Input: part model. Units: mm. Frame: model coordinates. A direction names the side the tool comes from. Round coordinates to 2 decimals unless told otherwise and drop trailing zeros. Loops run counter-clockwise (first coordinate to the right, second up) from the corner with the lowest first, then second, coordinate; pieces in that order, holes last.
(1) First-contact query: pin 1 Ø10 at (x, z) = (22.5, -40) entering from -Y. Flat tip, straight axial feed; report the tip coordinate or a pass-through.
(2) Cut plane B-B, the plane x = 22.5. Output: boundary loops of the cut face in (y, z).
(3) Draft query along Z for faces 1 (the face through (-97.5, -9, 1)), 2 (the face through (27.58, -8.88, -2.11)). Return one class per face: released by +Z, released by -Z, zero draft, split by the parting line, or undercut.
(4) Line query: line 1 (Z direction, x = -20, y = -7); line 2 (Z direction, x = 22.5, y = -6.5); line 3 (X direction, y = -16, z = -42). Output: solid intervals per line, ascending.
(5) Cut plane A-A, the plane z = 40. Give the number of separate pieces and of enclosed holes in the cut face, and give its area (3 significant figures).
(6) Cut plane C-C, the plane x = -80. Output: boundary loops of the cut face in (y, z).
(7) Access query for faces 3 (the face through (77, -9, -40)), 4 (the face through (45, -9, 42)). Directions: +Z, -Z, +X, -X, +Y, -Y. A direction counts if a zero-diameter tool reaches every point of the face in a straight line with its end or side. Return the directions, or none.
from build123d import *

# Parameters (mm, degrees)
F0_R     = 5.5
F0_W     = 30
F0_H     = 59.6731263399
F0_H_2   = 20
F1_DEPTH = 18
F2_SIZE  = 0.5
F3_W     = 30
F3_H     = 79.6731263399
F4_DEPTH = 25


with BuildPart() as f1:
    # F0 (on Front) → F1 (new body)
    with BuildSketch(Plane.XZ):
        Polygon((-97.5, 52.5), (-97.5, -52.5), (97.5, -52.5), (97.5, 52.5), (45, 52.5), (45, 32.5), (15, 32.5), (15, 52.5), align=None)
        with Locations((-80, -40)):
            Circle(F0_R, mode=Mode.SUBTRACT)
        with Locations((-20, -40)):
            Circle(F0_R, mode=Mode.SUBTRACT)
        with Locations((-80, 0)):
            Circle(F0_R, mode=Mode.SUBTRACT)
        with Locations((-20, 0)):
            Circle(F0_R, mode=Mode.SUBTRACT)
        with Locations((22.5, -40)):
            Circle(F0_R, mode=Mode.SUBTRACT)
        with Locations((82.5, -40)):
            Circle(F0_R, mode=Mode.SUBTRACT)
        with Locations((22.5, 0)):
            Circle(F0_R, mode=Mode.SUBTRACT)
        with Locations((82.5, 0)):
            Circle(F0_R, mode=Mode.SUBTRACT)
        with Locations((-80, 40)):
            Circle(F0_R, mode=Mode.SUBTRACT)
        with Locations((-20, 40)):
            Circle(F0_R, mode=Mode.SUBTRACT)
        with Locations((82.5, 40)):
            Circle(F0_R, mode=Mode.SUBTRACT)
        with Locations((30, 82.33656317)):
            Rectangle(F0_W, F0_H)
        with Locations((30, 42.5)):
            Rectangle(F0_W, F0_H_2)
    extrude(amount=F1_DEPTH)

    # F2
    f2_edges = [f1.edges().sort_by_distance(p)[0] for p in [
        (-74.5, -9, 40),
        (-85.5, 0, 40),
        (-85.5, -18, 40),
        (-74.5, -9, 0),
        (-85.5, 0, 0),
        (-85.5, -18, 0),
        (-74.5, -9, -40),
        (-85.5, 0, -40),
        (-85.5, -18, -40),
        (-14.5, -9, 40),
        (-25.5, 0, 40),
        (-25.5, -18, 40),
        (-14.5, -9, 0),
        (-25.5, 0, 0),
        (-25.5, -18, 0),
        (-14.5, -9, -40),
        (-25.5, 0, -40),
        (-25.5, -18, -40),
        (28, -9, 0),
        (17, 0, 0),
        (17, -18, 0),
        (28, -9, -40),
        (17, 0, -40),
        (17, -18, -40),
        (88, -9, 40),
        (77, 0, 40),
        (77, -18, 40),
        (88, -9, 0),
        (77, 0, 0),
        (77, -18, 0),
        (88, -9, -40),
        (77, 0, -40),
        (77, -18, -40),
    ]]
    chamfer(f2_edges, length=F2_SIZE)

    # F3 (on face) → F4 (cut)
    with BuildSketch(Plane.XZ.offset(18)):
        with Locations((30, 72.33656317)):
            Rectangle(F3_W, F3_H)
    extrude(amount=-F4_DEPTH, mode=Mode.SUBTRACT)


solid = f1.part
Reported:
1. pin 1: passes through
2. outline: (-18, -52.5) - (0, -52.5) - (0, -46) - (-0.5, -45.5) - (-17.5, -45.5) - (-18, -46) - close; (-18, -34) - (-17.5, -34.5) - (-0.5, -34.5) - (0, -34) - (0, -6) - (-0.5, -5.5) - (-17.5, -5.5) - (-18, -6) - close; (-18, 6) - (-17.5, 5.5) - (-0.5, 5.5) - (0, 6) - (0, 32.5) - (-18, 32.5) - close
3. face 1: zero draft
3. face 2: undercut
4. line 1: z = -52.5 to -45.5, -34.5 to -5.5, 5.5 to 34.5, 45.5 to 52.5
4. line 2: z = -52.5 to -45.5, -34.5 to -5.5, 5.5 to 32.5
4. line 3: x = -97.5 to -85.12, -74.88 to -25.12, -14.88 to 17.38, 27.62 to 77.38, 87.62 to 97.5
5. separate pieces: 5
5. enclosed holes: 0
5. area: 2,370 mm2
6. outline: (-18, -52.5) - (0, -52.5) - (0, -46) - (-0.5, -45.5) - (-17.5, -45.5) - (-18, -46) - close; (-18, -34) - (-17.5, -34.5) - (-0.5, -34.5) - (0, -34) - (0, -6) - (-0.5, -5.5) - (-17.5, -5.5) - (-18, -6) - close; (-18, 6) - (-17.5, 5.5) - (-0.5, 5.5) - (0, 6) - (0, 34) - (-0.5, 34.5) - (-17.5, 34.5) - (-18, 34) - close; (-18, 46) - (-17.5, 45.5) - (-0.5, 45.5) - (0, 46) - (0, 52.5) - (-18, 52.5) - close
7. face 3: +Y, -Y
7. face 4: +Z, +Y, -Y
